Can you work these out from the model? Positions are in its coordinate system, mm. Face numbers are marked on the shaded views. A direction names the side the tool comes from. Give positions to 0.01 mm unless a question says otherwise; leave off trailing zeros. Write each loop counter-clockwise with the first axis right and the second up, starting at its lowest first coordinate (ties: lowest second). Pieces come first, ordered by that corner, then holes. Notation, with made-up numbers: (1.25, 71) -> (41.25, 71) arc R28 ccw to (41.25, 104) -> close; hole circle Ø7 at (65, -3.5). An arc over 180 degrees is marked (long way). One line per item, written item: value.
from build123d import *

# Parameters (mm, degrees)
SKETCH1_W           = 63.5
SKETCH1_H           = 127
BOSS_EXTRUDE1_DEPTH = 6.35
SKETCH2_R           = 1.5875
CUT_EXTRUDE1_DEPTH  = 143.132235964
SKETCH3_W           = 63.5
SKETCH3_H           = 6.35
BOSS_EXTRUDE2_DEPTH = 38.1
CUT_EXTRUDE2_DEPTH  = 144.403190341


with BuildPart() as part:
    # Sketch1 → Boss-Extrude1 (new body)
    with BuildSketch(Plane.XY):
        with Locations((31.75, 63.5)):
            Rectangle(SKETCH1_W, SKETCH1_H)
    extrude(amount=BOSS_EXTRUDE1_DEPTH)

    # Sketch2 → Cut-Extrude1 (cut, through all)
    with BuildSketch(Plane.XY.offset(6.35)):
        with Locations((55.88, 61.595)):
            Circle(SKETCH2_R)
        with Locations((7.62, 62.865)):
            Circle(SKETCH2_R)
        with Locations((20.32, 113.665)):
            Circle(SKETCH2_R)
        with Locations((48.26, 113.665)):
            Circle(SKETCH2_R)
    extrude(amount=-CUT_EXTRUDE1_DEPTH, mode=Mode.SUBTRACT)

    # Sketch3 → Boss-Extrude2 (add)
    with BuildSketch(Plane.XY.offset(6.35)):
        with Locations((31.75, 3.175)):
            Rectangle(SKETCH3_W, SKETCH3_H)
    extrude(amount=BOSS_EXTRUDE2_DEPTH)

    # Sketch4 → Cut-Extrude2 (cut, through all)
    with BuildSketch(Plane(origin=(0, 6.35, 0), x_dir=(1, 0, 0), z_dir=(0, 1, 0))):
        with BuildLine():
            Line((13.716, -28.194), (49.784, -28.194))
            ThreePointArc((49.784, -28.194), (53.34, -31.75), (49.784, -35.306))
            Line((49.784, -35.306), (13.716, -35.306))
            ThreePointArc((13.716, -35.306), (10.16, -31.75), (13.716, -28.194))
        make_face()
    extrude(amount=-CUT_EXTRUDE2_DEPTH, mode=Mode.SUBTRACT)


solid = part.part
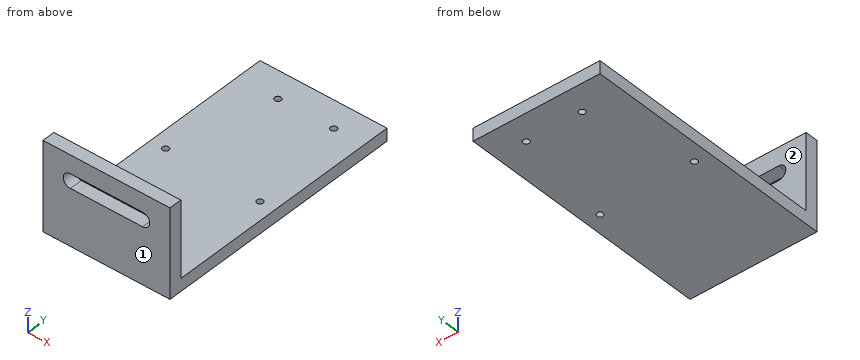
1) If we section it at B-B (z = 31.75): Write out the boundary of the cut face in (x, y).
Answer list:
outline: (0, 0) -> (10.16, 0) -> (10.16, 6.35) -> (0, 6.35) -> close; (53.34, 0) -> (63.5, 0) -> (63.5, 6.35) -> (53.34, 6.35) -> close
2) Will these pins go through, and if not, where does the flat tip stop? pin 1 (4 mm diameter, centred on x = 30.5, z = 6.5, fed in from +Y); pin 2 (19 mm diameter, centred on x = 37.5, z = 20.5, fed in from +Y); pin 3 (12 mm diameter, centred on x = 42, y = 107, fed in from +Z); pin 4 (2.5 mm diameter, centred on x = 48.26, y = 113.665, fed in from +Z).
Answer list:
pin 1: stops at y = 127
pin 2: stops at y = 6.35
pin 3: stops at z = 6.35
pin 4: passes through
3) For the marked faces 1 and 2, which set-ups out of +Z, -Z, +X, -X, +Y, -Y let a thin tool reach every point of the face, with its end or its side?
Answer list:
face 1: +Z, -Z, +X, -X, -Y
face 2: +Z, +X, -X, +Y
4) If we section it at A-A (x = 7.62): Write out the boundary of the cut face in (y, z), and give its area (3 significant figures).
Answer list:
outline: (0, 0) -> (61.28, 0) -> (61.28, 6.35) -> (6.35, 6.35) -> (6.35, 44.45) -> (0, 44.45) -> close; (64.45, 0) -> (127, 0) -> (127, 6.35) -> (64.45, 6.35) -> close
area: 1,030 mm^2
5) If we section it at D-D (x = 35.5): Write out the boundary of the cut face in (y, z).
Answer list:
outline: (0, 0) -> (127, 0) -> (127, 6.35) -> (6.35, 6.35) -> (6.35, 28.19) -> (0, 28.19) -> close; (0, 35.31) -> (6.35, 35.31) -> (6.35, 44.45) -> (0, 44.45) -> close
6) If we section it at C-C (x = 20.32): Write out the boundary of the cut face in (y, z).
Answer list:
outline: (0, 0) -> (112.08, 0) -> (112.08, 6.35) -> (6.35, 6.35) -> (6.35, 28.19) -> (0, 28.19) -> close; (0, 35.31) -> (6.35, 35.31) -> (6.35, 44.45) -> (0, 44.45) -> close; (115.25, 0) -> (127, 0) -> (127, 6.35) -> (115.25, 6.35) -> close
7) I need wall thicknesses on L1, parallel to Y at x = 55.88, z = 2; L2, parallel to Z at x = 44, y = 5.5; L3, parallel to Y at x = 47, z = 39. Which ranges of each line are inside material? Lowest first, please.
Answer list:
L1: y = 0 to 60.01, 63.18 to 127
L2: z = 0 to 28.19, 35.31 to 44.45
L3: y = 0 to 6.35
